```python
from build123d import *

# Parameters (mm, degrees)
BOSS_EXTRUDE1_DEPTH = 5
FILLET1_R           = 5
SKETCH2_R           = 1.3
CUT_EXTRUDE1_DEPTH  = 10
BOSS_EXTRUDE2_DEPTH = 35
BOSS_EXTRUDE3_DEPTH = 20
BOSS_EXTRUDE4_DEPTH = 6
BOSS_EXTRUDE5_START = 0.9
SKETCH6_R           = 4.9
SKETCH6_R_2         = 1.3
BOSS_EXTRUDE5_DEPTH = 0.9


with BuildPart() as part:
    # Sketch1 → Boss-Extrude1 (new body)
    with BuildSketch(Plane(origin=(0, 0, 0), x_dir=(1, 0, 0), z_dir=(0, 1, 0))):
        Polygon((4.09199016, 5.61187779), (0, 10), (0, 1.796035233), align=None)
        Polygon((0, 1.796035233), (0, 10), (-36.567685081, -24.099918003), (-32.475694921, -28.488040213), (-1.926011986, 0), align=None)
        Polygon((42, 10), (0, 10), (4.09199016, 5.61187779), (0, 1.796035233), (0, 0), (42, 0), align=None)
        Polygon((0, 0), (0, 1.796035233), (-1.926011986, 0), align=None)
    extrude(amount=BOSS_EXTRUDE1_DEPTH)

    # Fillet1
    fillet1_edges = [part.edges().sort_by_distance(p)[0] for p in [
        (42, 2.5, 0),
        (42, 2.5, -10),
    ]]
    fillet(fillet1_edges, radius=FILLET1_R - 0.0001)  # a hair under: the kernel refuses the full size

    # Sketch2 → Cut-Extrude1 (cut)
    with BuildSketch(Plane(origin=(0, 5, 0), x_dir=(1, 0, 0), z_dir=(0, 1, 0))):
        with Locations(Location((37, 5, 0), (0, 0, 270))):
            Circle(SKETCH2_R)
    extrude(amount=-CUT_EXTRUDE1_DEPTH, mode=Mode.SUBTRACT)

    # Sketch3 → Boss-Extrude2 (add)
    with BuildSketch(Plane(origin=(0, 5, 0), x_dir=(1, 0, 0), z_dir=(0, 1, 0))):
        Polygon((-36.567685081, -24.099918003), (-32.475694921, -28.488040213), (-17.200853453, -14.244020106), (-21.292843614, -9.855897897), align=None)
    extrude(amount=BOSS_EXTRUDE2_DEPTH)

    # Sketch4 → Boss-Extrude3 (add)
    with BuildSketch(Plane.XZ):
        Polygon((-36.567685081, 24.099918003), (-32.475694921, 28.488040213), (-17.200853453, 14.244020106), (-21.292843614, 9.855897897), align=None)
    extrude(amount=BOSS_EXTRUDE3_DEPTH)

    # Sketch5 → Boss-Extrude4 (add)
    with BuildSketch(Plane(origin=(-4.987820251, 0, -5.348782369), x_dir=(-0.7313537016191739, 0, 0.6819983600624947), z_dir=(-0.6819983600624948, 0, -0.731353701619174))):
        Polygon((22.294306197, -20), (22.294306197, 0), (9.326364945, 0), align=None)
        Polygon((9.326364945, 5), (22.294306197, 40), (22.294306197, 5), align=None)
    extrude(amount=-BOSS_EXTRUDE4_DEPTH)

    # Sketch6 → Boss-Extrude5 (add)
    with BuildSketch(Plane(origin=(0, 5, 0), x_dir=(1, 0, 0), z_dir=(0, 1, 0)).offset(BOSS_EXTRUDE5_START)):
        with Locations(Location((37, 5, 0), (0, 0, 270))):
            Circle(SKETCH6_R)
        with Locations(Location((37, 5, 0), (0, 0, 270))):
            Circle(SKETCH6_R_2, mode=Mode.SUBTRACT)
    extrude(amount=-BOSS_EXTRUDE5_DEPTH)


solid = part.part
```
The listing builds one solid part. Answer for the finished solid, in the listing's coordinates (mm). A direction names the side the tool comes from. Give positions to 0.01 mm unless a question says otherwise; leave off trailing zeros. Loops run counter-clockwise (first coordinate to the right, second up) from the corner with the lowest first, then second, coordinate; pieces in that order, holes last. Notation, with made-up numbers: M -28,47.5 L 3,47.5 A24 ccw 3,76.5 Z; hole C -27.5,26.5 d8. An arc over 180 degrees is marked long. One line per item, written item: value.
1. For faces 4 (the face through (-34.55, 10.42, 26.263)), 5 (the face through (34.02, 5.46, -8.89)), determine the directions among +Z, -Z, +X, -X, +Y, -Y from which every point of the face is accessible in a straight line to the end or side of a thin tool.
Found:
face 4: +Z, -X, +Y, -Y
face 5: +Y
2. For a pull along Z with two mould halves and no side action, classify faces 1 (the face through (17, 2, 0)), 2 (the face through (38.29, 2.99, -5.17)), 3 (the face through (19, 2, -10)) as pulls with the +Z half, pulls with the -Z half, needs draft (parallel to the pull), parting line crosses it, or undercut.
Found:
face 1: pulls with the +Z half
face 2: undercut
face 3: pulls with the -Z half
3. Section D-D on x = 33.5 is taken. Determine the outline of the cut face in (y, z), plus the area to 3 significant figures.
Found:
outline: M 0,-10 L 5,-10 L 5,-8.43 L 5.9,-8.43 L 5.9,-1.57 L 5,-1.57 L 5,0 L 0,0 Z
area: 56.2 mm^2
4. Each of these flat-tipped pins is pushed along its axis until it touches: P1, Ø6, axis at x = -1, z = 0, coming from the -Y side; P2, Ø12, axis at x = -16, z = 18, coming from the -Y side; P3, Ø17, axis at x = 18.5, z = -0.5, coming from the +Y side; P4, Ø3, axis at x = 35, z = -5, coming from the +Y side. Where does it stop, or does it pass through?
Found:
P1: y = 0
P2: y = -20
P3: y = 5
P4: y = 5.9
5. Find the intervals of material crossed by probe 1 along Y at (x, z) = (-0.5, -7.5); probe 2 along X at (y, z) = (3, -5); probe 3 along Z at (x, y) = (-24.5, 10.5), in increasing order.
Found:
probe 1: 0 to 5
probe 2: -5.36 to 35.7, 38.3 to 42
probe 3: 12.85 to 21.05
6. Section B-B on x = -14.5 is taken. Determine the outline of the cut face in (y, z), plus the area to 3 significant figures.
Found:
outline: M -14.3,11.73 L -5.68,3.52 L 14.93,3.52 L 30.03,11.73 Z
area: 266 mm^2
7. Section A-A on y = 36 is taken. Determine the outline of the cut face in (x, z), plus the area to 3 significant figures.
Found:
outline: M -36.57,24.1 L -20.21,8.85 L -16.12,13.23 L -32.48,28.49 Z
area: 134 mm^2
8. Section C-C on z = 16.5 is taken. Determine the outline of the cut face in (x, y).
Found:
outline: M -28.42,-20 L -19.62,-20 L -19.62,40 L -28.42,40 Z
